from build123d import *

# Parameters (mm, degrees)
SALIENTE_EXTRUIR1_DEPTH = 5
CROQUIS2_R              = 3
SALIENTE_EXTRUIR2_DEPTH = 8
CHAFL_N1_SIZE           = 0.5
CROQUIS3_R              = 2
CORTAR_EXTRUIR1_DEPTH   = 17.9
CROQUIS4_R              = 3.45
CORTAR_EXTRUIR2_DEPTH   = 6.5
CORTAR_EXTRUIR3_DEPTH   = 11
CHAFL_N2_SIZE           = 0.5
CHAFL_N3_SIZE           = 1.2
SALIENTE_EXTRUIR3_START = -1
CROQUIS6_R              = 4.25
CROQUIS6_R_2            = 3.45
SALIENTE_EXTRUIR3_DEPTH = 4.8


with BuildPart() as part:
    # Croquis1 → Saliente-Extruir1 (new body, symmetric)
    with BuildSketch(Plane.XY):
        Polygon((0, 4), (-2.1, 4), (-2.1, 8.4), (-4.5, 8.4), (-8.9, 4), (-8.9, -4), (-4.5, -8.4), (-2.1, -8.4), (-2.1, -4), (0, -4), align=None)
    extrude(amount=SALIENTE_EXTRUIR1_DEPTH, both=True)

    # Croquis2 → Saliente-Extruir2 (add)
    with BuildSketch(Plane(origin=(0, 0, 0), x_dir=(0, 0, -1), z_dir=(1, 0, 0))):
        Circle(CROQUIS2_R)
    extrude(amount=SALIENTE_EXTRUIR2_DEPTH)

    # Chaflán1
    chafl_n1_edges = [part.edges().sort_by_distance(p)[0] for p in [
        (0, 0, 3),
        (8, 0, 3),
    ]]
    chamfer(chafl_n1_edges, length=CHAFL_N1_SIZE)

    # Croquis3 → Cortar-Extruir1 (cut, through all)
    with BuildSketch(Plane(origin=(8, 0, 0), x_dir=(0, 0, -1), z_dir=(1, 0, 0))):
        Circle(CROQUIS3_R)
    extrude(amount=-CORTAR_EXTRUIR1_DEPTH, mode=Mode.SUBTRACT)

    # Croquis4 → Cortar-Extruir2 (cut)
    with BuildSketch(Plane.ZY.offset(8.9)):
        Circle(CROQUIS4_R)
    extrude(amount=-CORTAR_EXTRUIR2_DEPTH, mode=Mode.SUBTRACT)

    # Croquis5 → Cortar-Extruir3 (cut, through all)
    with BuildSketch(Plane.XY.offset(5)):
        Polygon((-3.1, 7.2), (-3.1, -7.2), (-4.002943725, -7.2), (-7.7, -3.502943725), (-7.7, 3.502943725), (-4.002943725, 7.2), align=None)
    extrude(amount=-CORTAR_EXTRUIR3_DEPTH, mode=Mode.SUBTRACT)

    # Chaflán2
    chafl_n2_edges = [part.edges().sort_by_distance(p)[0] for p in [
        (-1.05, -4, -5),
        (-2.1, -6.2, -5),
        (-3.3, -8.4, -5),
        (-6.7, -6.2, -5),
        (-6.7, 6.2, -5),
        (-3.3, 8.4, -5),
        (-2.1, 6.2, 5),
        (-2.1, 6.2, -5),
        (-1.05, 4, -5),
        (-3.3, 8.4, 5),
        (-6.7, 6.2, 5),
        (-6.7, -6.2, 5),
        (-3.3, -8.4, 5),
        (-2.1, -6.2, 5),
        (-1.05, -4, 5),
        (-1.05, 4, 5),
    ]]
    chamfer(chafl_n2_edges, length=CHAFL_N2_SIZE)

    # Chaflán3
    chafl_n3_edges = [part.edges().sort_by_distance(p)[0] for p in [
        (-2.4, 0, 2),
    ]]
    chamfer(chafl_n3_edges, length=CHAFL_N3_SIZE)

    # Croquis6 → Saliente-Extruir3 (add)
    with BuildSketch(Plane.ZY.offset(8.9).offset(SALIENTE_EXTRUIR3_START)):
        Circle(CROQUIS6_R)
        Circle(CROQUIS6_R_2, mode=Mode.SUBTRACT)
    extrude(amount=-SALIENTE_EXTRUIR3_DEPTH)


solid = part.part
CAD build for the part. Positions are in the model's coordinates, mm. A direction names the side the tool comes from. Coordinates: 2 decimals unless noted, no trailing zeros. Loops run counter-clockwise (first coordinate to the right, second up) from the corner with the lowest first, then second, coordinate; pieces in that order, holes last. Notation, with made-up numbers: (79, 45.5) - (109, 45.5) arc R19 ccw to (109, 56.5) - close; hole circle Ø4 at (50.5, -13). An arc over 180 degrees is marked (long way). Write item = value, one per line. Start each with the question number.
Q1. Pull direction Y, two halves, no side cores. Call faces 1 (the flat face through (-3, -8.4, 0)), 2 (the flat face through (-7.7, 0, 4.6)), 3 (the flat face through (-2.8, 0.6, -5)): pulls with the +Y half, pulls with the -Y half, needs draft (parallel to the pull), parting line crosses it, or undercut.
Q2. Flat gauge pins, fed straight in: pin 1 Ø4 at (x, y) = (4.5, -1) entering from +Z; pin 2 Ø1.7 at (x, z) = (-1, 2) entering from +Y; pin 3 Ø1.3 at (y, z) = (6, -0.5) entering from +X; pin 4 Ø3.5 at (y, z) = (0, 0) entering from -X. Where does each tip first touch, or does it go through?
Q3. Drill centre lines: L1, parallel to Y at x = -5.5, z = 0; L2, parallel to X at y = 2.5, z = 3.5; L3, parallel to Y at x = -5.25, z = -1.75. Where is each one in solid material? Low to high.
Q4. Which spindle directions (+Z, -Z, +X, -X, +Y, -Y) get a long thin tool onto all of the face, cutting with end or side? Do faces 4 (the flat face through (-2.1, 6, 0)), 5 (the flat face through (0, -1.8, 3.4)), 6 (the flat face through (-1, -4, 0)), 7 (the flat face through (-7.7, 0, -4.5)), 8 (the cylindrical face through (-5.432, 4.214, -0.553)). Say none if no direction does.
Q5. Cut at D-D, the plane z = 4. List the corners of the cut face in (x, y).
Q6. Cut at A-A, the plane x = -5.25. List the corners of the cut face in (y, z), then the cut area to 3 significant figures.
Q7. Cut at C-C, the plane x = 7. List the corners of the cut face in (y, z).
Computed:
q1.face_1 = pulls with the -Y half
q1.face_2 = undercut
q1.face_3 = needs draft
q2.pin_1 = 3
q2.pin_2 = 4
q2.pin_3 = -2.1
q2.pin_4 = through
q3.L1 = -7.4 to -5.7, -4.25 to -3.45, 3.45 to 4.25, 5.7 to 7.4
q3.L2 = -8.9 to -7.7, -3.1 to 0
q3.L3 = -7.65 to -5.95, -3.87 to -2.97, 2.97 to 3.87, 5.95 to 7.65
q4.face_4 = +Z, -Z, +X, +Y
q4.face_5 = +X
q4.face_6 = +Z, -Z, +X, -Y
q4.face_7 = -Z
q4.face_8 = none
q5.outline = (-8.9, -4) - (-4.5, -8.4) - (-2.1, -8.4) - (-2.1, -4) - (0, -4) - (0, 4) - (-2.1, 4) - (-2.1, 8.4) - (-4.5, 8.4) - (-8.9, 4) - close; hole (-7.7, -3.5) - (-4, -7.2) - (-3.1, -7.2) - (-3.1, -1.44) - (-7.7, -1.44) - close; hole (-7.7, 1.44) - (-3.1, 1.44) - (-3.1, 7.2) - (-4, 7.2) - (-7.7, 3.5) - close
q6.outline = (-7.65, -4.5) - (-6.94, -5) - (-5.95, -5) - (-5.95, 5) - (-6.94, 5) - (-7.65, 4.5) - close; circle Ø8.5 at (0, 0); (5.95, -5) - (6.94, -5) - (7.65, -4.5) - (7.65, 4.5) - (6.94, 5) - (5.95, 5) - close; hole circle Ø6.9 at (0, 0)
q6.area = 52.6 mm²
q7.outline = circle Ø6 at (0, 0); hole circle Ø4 at (0, 0)
